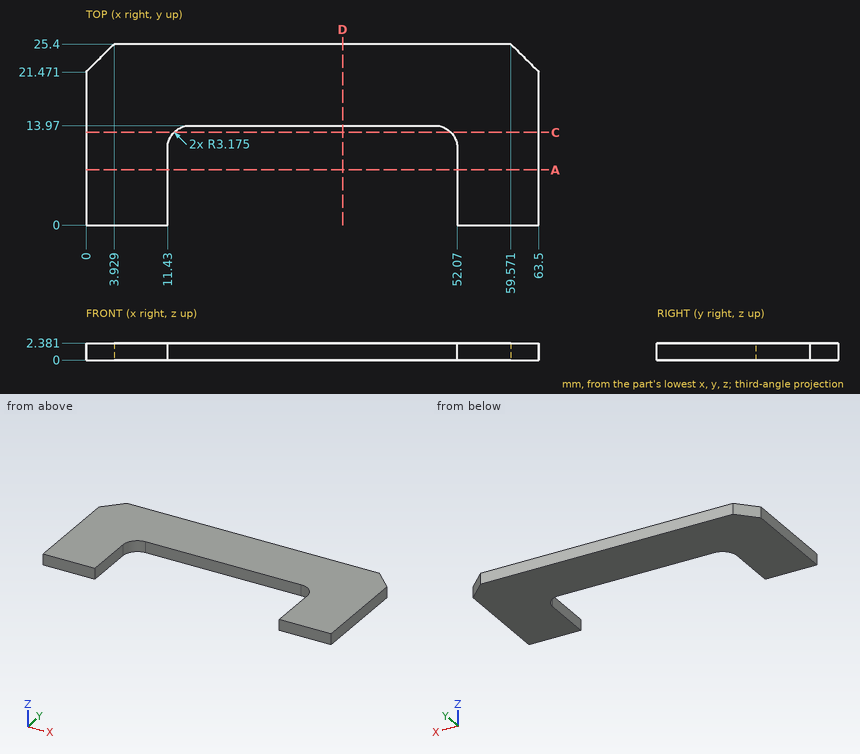
The figure shows three views and two pictorial views of one solid part (mm, origin at its lowest corner). Answer the questions. Give positions to 0.01 mm unless a question says otherwise; leave off trailing zeros. Order: outer loops, then holes, each group sorted by start corner. A loop starts at its lowest first (then second) coordinate and runs counter-clockwise, first axis right, second up. Notation, with made-up numbers: (66, 24.5) -> (73, 24.5) arc R31 cw to (73, 53.5) -> close; hole circle Ø3 at (14, 48). An arc over 180 degrees is marked (long way). Answer as a JSON object with one key per item and string values. Group by question number.
Item 1: The part is cut by section C-C on y = 13. Write down the section's boundary in (x, z).
Item 2: Flat-ended cylindrical pins translate along their axes: pin 1 (1.2 mm diameter, centred on x = 30, z = 0.5, fed in from -Y); pin 2 (1.5 mm diameter, centred on x = 52, y = 4, fed in from +Z); pin 3 (1 mm diameter, centred on x = 51, z = 1, fed in from -Y). Find the tip coordinate at first contact, or state that the pin passes through.
Item 3: Consider L1, parallel to X at y = 2.25, z = 1.3; L2, parallel to X at y = 12.25, z = 1.35; L3, parallel to Y at x = 18, z = 1.35. Determine where each line is inside the solid, lowest interval first. Write a range as from..to.
Item 4: The part is cut by section A-A on y = 7.75. Write down the section's boundary in (x, z).
Item 5: The part is cut by section D-D on x = 36. Write down the section's boundary in (y, z).
Result set:
{
 "1": {"outline": "(0, 0) -> (12.32, 0) -> (12.32, 2.38) -> (0, 2.38) -> close; (51.18, 0) -> (63.5, 0) -> (63.5, 2.38) -> (51.18, 2.38) -> close"},
 "2": {"pin 1": "y = 13.97", "pin 2": "z = 2.38", "pin 3": "y = 12.61"},
 "3": {"L1": "0..11.43, 52.07..63.5", "L2": "0..11.78, 51.72..63.5", "L3": "13.97..25.4"},
 "4": {"outline": "(0, 0) -> (11.43, 0) -> (11.43, 2.38) -> (0, 2.38) -> close; (52.07, 0) -> (63.5, 0) -> (63.5, 2.38) -> (52.07, 2.38) -> close"},
 "5": {"outline": "(13.97, 0) -> (25.4, 0) -> (25.4, 2.38) -> (13.97, 2.38) -> close"}
}
